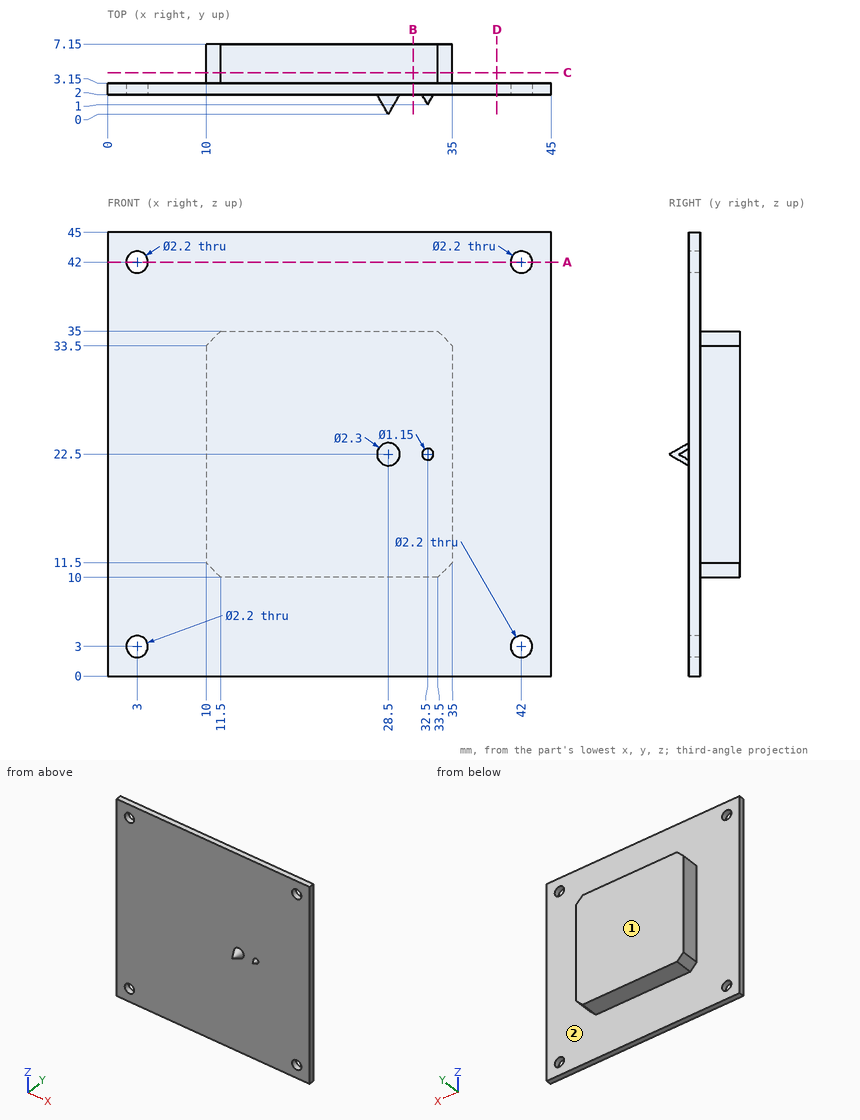
Here's the drawing with two shaded views (mm, measured from the low corner). I have some questions. A direction names the side the tool comes from. Give positions to 0.01 mm unless a question says otherwise; leave off trailing zeros. Loops run counter-clockwise (first coordinate to the right, second up) from the corner with the lowest first, then second, coordinate; pieces in that order, holes last. Notation, with made-up numbers: M 83.5,-7 L 115.5,-7 A10 ccw 115.5,9 Z; hole C 44.5,88.5 d5. An arc over 180 degrees is marked long. One line per item, written item: value. Start each with the question number.
1) If we section it at C-C, the plane y = 4.25: Write out the boundary of the cut face in (x, z), and give its area (4 significant figures).
2) If we section it at A-A, the plane z = 42: Write out the boundary of the cut face in (x, y).
3) If we section it at D-D, the plane x = 39.5: Write out the boundary of the cut face in (y, z).
4) I'm going to push flat-ended pins straight in: pin 1 (3 mm diameter, centred on x = 3, z = 3, fed in from +Y); pin 2 (5 mm diameter, centred on x = 6.5, z = 34.5, fed in from -Y); pin 3 (1.3 mm diameter, centred on x = 42, z = 42, fed in from -Y); pin 4 (2 mm diameter, centred on x = 20, y = 6, fed in from +Z). Where does each tip first touch, or does it pass through?
5) If I drill on line 1 (Z direction, x = 3, y = 2.6); line 2 (Y direction, x = 43.5, z = 6.5), over which ranges is the centre line in solid material (lowest first)? Write a range as [from, to].
6) If we section it at B-B, the plane x = 31: Write out the boundary of the cut face in (y, z), and give its area (3 significant figures).
7) On a 3-axis mill with a long thin cutter (end or side, diameter ignored), from which of +Z, -Z, +X, -X, +Y, -Y can I reach the whole of each face in a straight line? I mean the marked faces 1 and 2. Say none if no direction works.
Completed:
1. outline: M 10,11.5 L 11.5,10 L 33.5,10 L 35,11.5 L 35,33.5 L 33.5,35 L 11.5,35 L 10,33.5 Z
1. area: 620.5 mm^2
2. outline: M 0,2 L 1.9,2 L 1.9,3.15 L 0,3.15 Z; M 4.1,2 L 40.9,2 L 40.9,3.15 L 4.1,3.15 Z; M 43.1,2 L 45,2 L 45,3.15 L 43.1,3.15 Z
3. outline: M 2,0 L 3.15,0 L 3.15,45 L 2,45 Z
4. pin 1: stops at y = 3.15
4. pin 2: stops at y = 2
4. pin 3: passes through
4. pin 4: stops at z = 35
5. line 1: z = [0, 1.9], [4.1, 40.9], [43.1, 45]
5. line 2: y = [2, 3.15]
6. outline: M 2,0 L 3.15,0 L 3.15,10 L 7.15,10 L 7.15,35 L 3.15,35 L 3.15,45 L 2,45 Z
6. area: 152 mm^2
7. face 1: +Z, -Z, +X, -X, +Y
7. face 2: +Y
